Check sheet for the drawn part. Datum: minimum x, y, z corner. Units: mm. Round coordinates to 2 decimals unless told otherwise and drop trailing zeros. Write each loop counter-clockwise with the first axis right and the second up, starting at its lowest first coordinate (ties: lowest second). Pieces come first, ordered by that corner, then holes. Notation, with made-up numbers: (12.25, -1.75) - (70.25, -1.75) arc R16 ccw to (70.25, 6.25) - close; hole circle Ø2 at (81.25, 44). An arc over 180 degrees is marked (long way). Answer as a JSON object with one key per item and string values. Group by question number.
Item 1: Sectioned sample at D-D on z = 7. Record the boundary of the cut face in (x, y).
Item 2: Thickness scan on line 1 (X direction, y = 8.25, z = 5.25); line 2 (Z direction, x = 58.25, y = 8.25); line 3 (Z direction, x = 43, y = 7). Record the ranges inside material, lowest first.
Item 3: Sectioned sample at B-B on x = 22. Record the boundary of the cut face in (y, z), plus the area to 3 significant figures.
Item 4: Sectioned sample at A-A on y = 2. Record the boundary of the cut face in (x, z).
Item 5: Gauge pin test, flat ends, axial feed: P1, Ø1.1, axis at x = 21, y = 11, coming from the +Z side; P2, Ø3, axis at x = 20.5, y = 9, coming from the -Z side; P3, Ø1, axis at x = 6.5, z = 1.5, coming from the -Y side. Record the tip position at first contact, or that the pin passes through.
Item 6: Sectioned sample at C-C on y = 7.5. Record the boundary of the cut face in (x, z), plus the area to 3 significant figures.
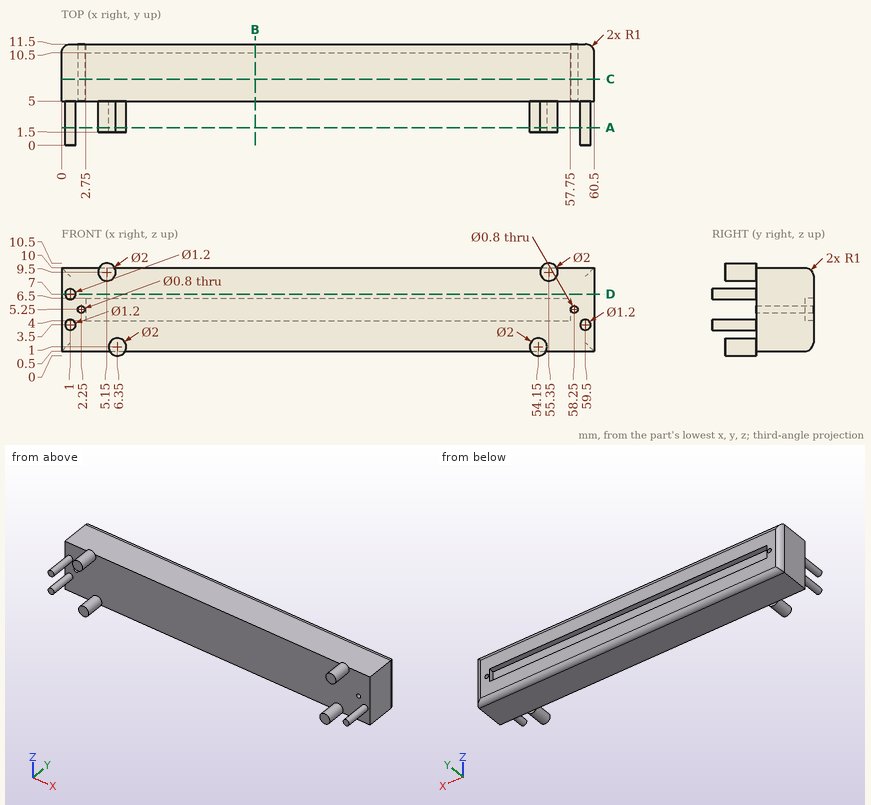
Completed:
{
 "1": {"outline": "(0, 5) - (0.4, 5) - (0.4, 0) - (1.6, 0) - (1.6, 5) - (60.5, 5) - (60.5, 10.5) arc R1 ccw to (59.5, 11.5) - (1, 11.5) arc R1 ccw to (0, 10.5) - close"},
 "2": {"line 1": "0 to 1.85, 2.65 to 57.85, 58.65 to 60.5", "line 2": "0.5 to 4.85, 5.65 to 10", "line 3": "0.5 to 10"},
 "3": {"outline": "(5, 0.5) - (10.5, 0.5) arc R1 ccw to (11.5, 1.5) - (11.5, 4) - (10.5, 4) - (10.5, 6.5) - (11.5, 6.5) - (11.5, 9) arc R1 ccw to (10.5, 10) - (5, 10) - close", "area": "58.8 mm²"},
 "4": {"outline": "circle Ø1.2 at (1, 3.5); circle Ø1.2 at (1, 7); circle Ø2 at (5.15, 9.5); circle Ø2 at (6.35, 1); circle Ø2 at (54.15, 1); circle Ø2 at (55.35, 9.5); circle Ø1.2 at (59.5, 3.5)"},
 "5": {"P1": "z = 10", "P2": "z = 0.5", "P3": "y = 1.5"},
 "6": {"outline": "(0, 0.5) - (60.5, 0.5) - (60.5, 10) - (0, 10) - close; hole circle Ø0.8 at (2.25, 5.25); hole circle Ø0.8 at (58.25, 5.25)", "area": "574 mm²"}
}
